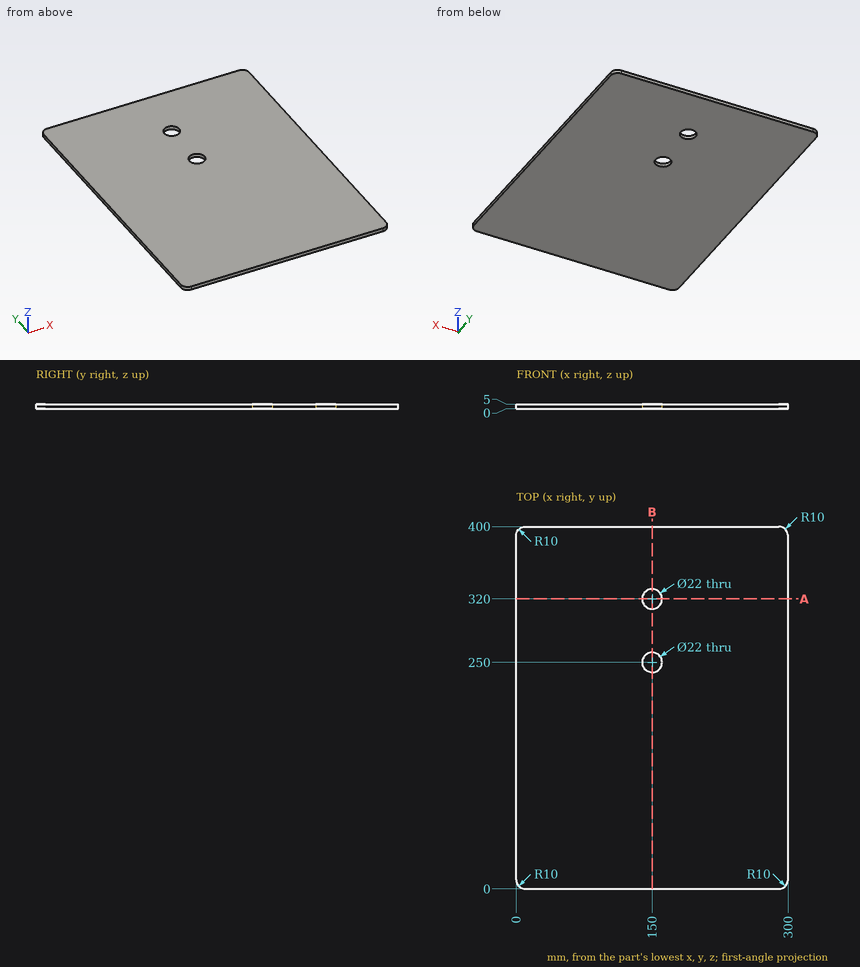
Geometry check sheet. Reference: drawing and pictorial views, mm from the part's lowest x, y, z. Coordinates: 2 decimals unless noted, no trailing zeros. Order: outer loops, then holes, each group sorted by start corner. A loop starts at its lowest first (then second) coordinate and runs counter-clockwise, first axis right, second up.
Item 1: Section check B-B, the plane x = 150. Enter the section's corners in (y, z), then the cut area to 3 significant figures.
Filled in:
outline: (0, 0) - (239, 0) - (239, 5) - (0, 5) - close; (261, 0) - (309, 0) - (309, 5) - (261, 5) - close; (331, 0) - (400, 0) - (400, 5) - (331, 5) - close
area: 1,780 mm2
Item 2: Material ranges on L1, parallel to Y at x = 150, z = 1.05; L2, parallel to X at y = 251, z = 1.05; L3, parallel to X at y = 255, z = 4.35, recorded low to high.
Filled in:
L1: y = 0 to 239, 261 to 309, 331 to 400
L2: x = 0 to 139.05, 160.95 to 300
L3: x = 0 to 140.2, 159.8 to 300
Item 3: Section check A-A, the plane y = 320. Enter the section's corners in (x, z).
Filled in:
outline: (0, 0) - (139, 0) - (139, 5) - (0, 5) - close; (161, 0) - (300, 0) - (300, 5) - (161, 5) - close
